```python
from build123d import *

# Parameters (mm, degrees)
EXTRUDE_1_DEPTH     = 5
SKETCH_2_R          = 1.5
CUT_EXTRUDE_1_DEPTH = 10
CUT_EXTRUDE_START   = -10
SKETCH_3_R          = 1.5
CUT_EXTRUDE_2_DEPTH = 10
SKETCH_4_R          = 1.5
CUT_EXTRUDE_3_DEPTH = 10
SKETCH_5_R          = 1.5
CUT_EXTRUDE_4_DEPTH = 10


with BuildPart() as part:
    # 草图1 → 凸台-拉伸1 (new body)
    with BuildSketch(Plane.XY):
        Polygon((0, 0), (112, 0), (201, -105), (201, -115), (201, -125), (112, -230), (56, -230), (0, -230), (-89, -125), (-89, -115), (-89, -105), align=None)
        Polygon((4.632806625, -10), (107.367193375, -10), (191, -108.667917928), (191, -115), (191, -121.332082072), (107.367193375, -220), (56, -220), (4.632806625, -220), (-79, -121.332082072), (-79, -115), (-79, -108.667917928), align=None, mode=Mode.SUBTRACT)
    extrude(amount=EXTRUDE_1_DEPTH)

    # 草图2 → 切除-拉伸1 (cut)
    with BuildSketch(Plane(origin=(0, 0, 0), x_dir=(1, 0, 0), z_dir=(0, 1, 0))):
        with Locations(Location((5, -2.5, 0), (0, 0, 270))):
            Circle(SKETCH_2_R)
        with Locations(Location((107, -2.5, 0), (0, 0, 270))):
            Circle(SKETCH_2_R)
    extrude(amount=-CUT_EXTRUDE_1_DEPTH, mode=Mode.SUBTRACT)

    # 草图3 → 切除-拉伸2 (cut)
    with BuildSketch(Plane.XZ.offset(230).offset(CUT_EXTRUDE_START)):
        with Locations(Location((5, 2.5, 0), (0, 0, 90))):
            Circle(SKETCH_3_R)
        with Locations(Location((107, 2.5, 0), (0, 0, 90))):
            Circle(SKETCH_3_R)
    extrude(amount=CUT_EXTRUDE_2_DEPTH, mode=Mode.SUBTRACT)

    # 草图4 → 切除-拉伸3 (cut)
    with BuildSketch(Plane.ZY.offset(89)):
        with Locations((2.5, -115)):
            Circle(SKETCH_4_R)
    extrude(amount=-CUT_EXTRUDE_3_DEPTH, mode=Mode.SUBTRACT)

    # 草图5 → 切除-拉伸4 (cut)
    with BuildSketch(Plane(origin=(201, 0, 0), x_dir=(0, 0, -1), z_dir=(1, 0, 0)).offset(CUT_EXTRUDE_START)):
        with Locations(Location((-2.5, -115, 0), (0, 0, 180))):
            Circle(SKETCH_5_R)
    extrude(amount=CUT_EXTRUDE_4_DEPTH, mode=Mode.SUBTRACT)


solid = part.part
```
CAD build for the part. Positions are in the model's coordinates, mm. A direction names the side the tool comes from. Round coordinates to 2 decimals unless told otherwise and drop trailing zeros. Loops run counter-clockwise (first coordinate to the right, second up) from the corner with the lowest first, then second, coordinate; pieces in that order, holes last. Notation, with made-up numbers: M -32,-2.75 L 25,-2.75 A30 ccw 25,27.25 Z; hole C 5.5,84.5 d4. An arc over 180 degrees is marked long. Return JSON: item names as keys, results as strings. Group by question number.
(1) Wall check: probe 1 along Y at (x, z) = (22, 0.85); probe 2 along Z at (x, y) = (-85, -115); probe 3 along X at (y, z) = (-3.5, 2.5). Give the ranges that are in metal, low to high. Write a range as [from, to].
(2) Saw through at C-C, the plane y = -129.5. List the corners of the cut face in (x, z).
(3) Tool access for faces 4 (the flat face through (149.769, -169.975, 2.465)), 5 (the flat face through (132, -38, 5)): list every direction of +Z, -Z, +X, -X, +Y, -Y with a clear straight run to the whole face (end or side of a thin tool).
(4) Saw through at B-B, the plane z = 2.5. Give the number of separate pieces and of enclosed holes in the cut face, and give its area (3 significant figures).
(5) Drop flat-ended pins along their axis: P1, Ø1, axis at y = -206.5, z = 1, coming from the -X side; P2, Ø1.8, axis at x = 107, z = 2.5, coming from the +Y side; P3, Ø0.9, axis at x = 108, z = 2.5, coming from the -Y side. Give the stop position or say it passes through.
(6) Mould opens along X. For faces 1 (the flat face through (157.123, -176.765, 2.465)), 2 (the flat face through (-43.877, -178.235, 2.465)), 3 (the flat face through (-36.598, -171.357, 2.465)) say: +X half, -X half, draft (parallel to the pull), parting line (faces both ways), or undercut.
(7) Saw through at A-A, the plane x = 36.5. List the corners of the cut face in (y, z), and give its area (3 significant figures).
Answer list:
{
 "1": {"probe 1": "[-230, -220], [-10, 0]", "probe 2": "[0, 1], [4, 5]", "probe 3": "[-2.97, 3.5], [6.5, 105.5], [108.5, 114.97]"},
 "2": {"outline": "M -85.19,0 L -72.08,0 L -72.08,5 L -85.19,5 Z; M 184.08,0 L 197.19,0 L 197.19,5 L 184.08,5 Z"},
 "3": {"face 4": "+Z, -Z", "face 5": "+Z, +X, -X, +Y, -Y"},
 "4": {"separate pieces": "6", "enclosed holes": "0", "area": "7,630 mm2"},
 "5": {"P1": "x = -20.34", "P2": "y = -10", "P3": "y = -220"},
 "6": {"face 1": "+X half", "face 2": "-X half", "face 3": "undercut"},
 "7": {"outline": "M -230,0 L -220,0 L -220,5 L -230,5 Z; M -10,0 L 0,0 L 0,5 L -10,5 Z", "area": "100 mm2"}
}
